Can you work these out from the model? Positions are in its coordinate system, mm. A direction names the side the tool comes from. Round coordinates to 2 decimals unless told otherwise and drop trailing zeros. Write each loop counter-clockwise with the first axis right and the second up, starting at its lowest first coordinate (ties: lowest second). Pieces come first, ordered by that corner, then holes. Notation, with made-up numbers: M 11.25,-21 L 28.25,-21 A19 cw 28.25,-16 Z; hole C 70,8.25 d11. An arc over 180 degrees is marked long. Use one line per item in the form item = value. Start each with the question number.
Autodesk Inventor part; units mm, degrees
ref_plane "YZ Plane" through (0, 0, 0) normal (1, 0, 0) x (0, 1, 0)
ref_plane "XZ Plane" through (0, 0, 0) normal (0, 1, 0) x (-1, 0, 0)
ref_plane "XY Plane" through (0, 0, 0) normal (0, 0, 1) x (1, 0, 0)
sketch "Esquisse1" plane through (0, 0, 0) normal (0, 1, 0) x (-1, 0, 0)
  line L0 (57.9966, -37.2402) -> (57.9966, 37.7598)
  circle A0 centre (52.9966, 25.0001) radius 1.75
  circle A1 centre (52.9966, 15.0001) radius 1.75
  line L1 (67, 0.0502) -> (-72, 0.0502)
  circle A2 centre (43, 25.2598) radius 1.75
  circle A3 centre (43, 15.2598) radius 1.75
  circle A4 centre (52.9966, -24.8996) radius 1.75
  circle A5 centre (52.9966, -14.8996) radius 1.75
  circle A6 centre (43, -25.1593) radius 1.75
  circle A7 centre (43, -15.1593) radius 1.75
  line L2 (0, 58.3407) -> (0, -80.6593)
  circle A8 centre (5, 31.7598) radius 2.75
  circle A9 centre (5, 22.7598) radius 1.75
  circle A10 centre (15, 32.5) radius 1.75
  circle A11 centre (15, 22.5) radius 1.75
  circle A12 centre (25, 32.5) radius 1.75
  circle A13 centre (25, 22.5) radius 1.75
  circle A14 centre (35, 22.5) radius 1.75
  circle A15 centre (5, -31.6593) radius 2.75
  circle A16 centre (5, -22.6593) radius 1.75
  circle A17 centre (15, -32.3995) radius 1.75
  circle A18 centre (15, -22.3995) radius 1.75
  circle A19 centre (25, -32.3995) radius 1.75
  circle A20 centre (25, -22.3995) radius 1.75
  circle A21 centre (35, -22.3995) radius 1.75
  line L3 (58, 10) -> (48, 10)
  line L4 (48, 10) -> (48, -10)
  line L5 (48, -10) -> (58, -10)
  line L6 (58, -10) -> (58, 10)
  line L7 (58, 10) -> (48, -10)
  line L8 (48, 10) -> (58, -10)
  line L9 (57.9966, 37.7598) -> (0, 37.7598)
  line L10 (0, -38.4609) -> (57.9966, -38.4609)
  line L11 (57.9966, -38.4609) -> (57.9966, 37.7598)
  line L12 (57.9966, 37.7598) -> (0, 37.7598)
  line L13 (0, 37.7598) -> (0, -38.4609)
  circle A22 centre (30, 0.0502) radius 11
  line L14 (42.9966, -35.3694) -> (42.9966, -32.3694)
  line L15 (42.9966, -32.3694) -> (33, -32.3694)
  line L16 (42.9966, -32.3694) -> (33, -35.5523)
  line L17 (42.9966, -35.3694) -> (33, -32.3694)
  line L18 (33, -32.3694) -> (33, -35.5523)
  line L19 (33, -35.5523) -> (42.9966, -35.3694)
  line L20 (42.9966, 31.7598) -> (42.9966, 34.7598)
  line L21 (42.9966, 34.7598) -> (32.9966, 34.7598)
  line L22 (42.9966, 34.7598) -> (32.9966, 31.7598)
  line L23 (42.9966, 31.7598) -> (32.9966, 34.7598)
  line L24 (32.9966, 34.7598) -> (32.9966, 31.7598)
  line L25 (32.9966, 31.7598) -> (42.9966, 31.7598)
  point P0 (0, 0)
  point P1 (0, 0)
  point P2 (0, 0)
  point P3 (53, 0)
  point P4 (57.9966, -10)
  point P5 (57.9966, 10)
  point P6 (38.783, -33.8694)
  point P7 (42.5405, 34.5217)
  point P8 (42.9966, -33.8694)
  point P9 (42.9966, 33.2598)
  point P10 (37.9983, -35.4609)
  dimension "d3" = 3.5
  dimension "d4" = 3.5
  dimension "d7" = 10
  dimension "d9" = 3.5
  dimension "d10" = 3.5
  dimension "d12" = 10
  dimension "d13" = 10
  dimension "d16" = 5
  dimension "d17" = 5
  dimension "d19" = 5.5
  dimension "d20" = 3.5
  dimension "d21" = 3.5
  dimension "d22" = 3.5
  dimension "d23" = 3.5
  dimension "d24" = 3.5
  dimension "d26" = 3.5
  dimension "d27" = 5
  dimension "d28" = 5
  dimension "d31" = 10
  dimension "d32" = 10
  dimension "d33" = 10
  dimension "d35" = 10
  dimension "d36" = 10
  dimension "d38" = 10
  dimension "d40" = 10
  dimension "d70" = 9
  dimension "d72" = 5
  dimension "d73" = 6
  dimension "d77" = 22
  dimension "d80" = 139
  dimension "d81" = 75
  dimension "d83" = 15
  dimension "d85" = 3
  dimension "d86" = 15
  dimension "d87" = 3
  dimension "d115" = 30
extrude "Extrusion1" add sketch "Esquisse1" along normal blind 3 contours L8 L7 L1 L0 | L5 L7 L8 | L1 L7 L0 | L4 L1 L8 L7 | L8 L1 L7 | L7 L1 L8 L3 | L4 L8 L1
sketch "Esquisse4" plane through (0, 3, 0) normal (0, 1, 0) x (1, 0, 0)
  point P0 (0, 0)
sketch "Esquisse5" plane through (0, 0, 0) normal (0, -1, 0) x (1, 0, 0)
  point P0 (0, 0)
sketch "Esquisse6" plane through (0, 0, 0) normal (0, -1, 0) x (1, 0, 0)
  point P0 (0, 0)
sketch "Esquisse7" plane through (0, 0, 0) normal (0, -1, 0) x (1, 0, 0)
  point P0 (0, 0)
sketch "Esquisse8" plane through (0, 0, 0) normal (0, -1, 0) x (1, 0, 0)
  point P0 (0, 0)
extrude "Extrusion5" cut sketch "Esquisse1" along normal blind 3 contours L8 L7 L1 L0 | L5 L7 L8 | L1 L7 L0 | L4 L1 L8 L7 | L8 L1 L7 | L7 L1 L8 L3 | L4 L8 L1 | A22 L1 | L1 A22
extrude "Extrusion7" add sketch "Esquisse1" along normal blind 3 contours L11 L10 L2 L1 A22 L4 L5 L0 | L3 L4 L1 A22 L2 L9 L0 | L17 L16 L14 | L19 L16 L17 | L16 L17 L15 | L16 L18 L17 | L23 L22 L20 | L25 L22 L23 | L22 L23 L21 | L22 L24 L23
extrude "Extrusion8" add sketch "Esquisse1" along normal blind 10 contours L23 L22 L20 | L25 L22 L23 | L22 L23 L21 | L22 L24 L23
extrude "Extrusion9" add sketch "Esquisse1" along normal blind 10 contours L17 L16 L14 | L19 L16 L17 | L16 L17 L15 | L16 L18 L17
sketch "Esquisse10" plane through (-42.9966, 3, -35.3694) normal (-0.0183, 0, -0.9998) x (-0.9998, 0, 0.0183)
  line L0 (1.2831, 0) -> (1.2831, 7)
  line L1 (1.2831, 7) -> (-10, 0)
  line L2 (-43.046, 0) -> (14.9409, 0)
  line L3 (-9.9983, 7) -> (0, 7)
  line L4 (1.2831, 0) -> (-9.9983, 7)
  circle A0 centre (-4.3576, 3.5) radius 1.75
  point P0 (-42.3423, -3)
  dimension "d108" = 3.5
sketch "Esquisse11" plane through (-42.9966, 3, 34.7598) normal (0, 0, 1) x (1, 0, 0)
  line L0 (10, 0) -> (10, 7)
  line L1 (10, 7) -> (-0.0034, 0)
  line L2 (-1.7534, 0) -> (1.7466, 0)
  line L3 (42.9966, 0) -> (-15, 0)
  line L4 (0, 0) -> (0, 7)
  line L5 (10, 0) -> (0, 7)
  circle A0 centre (4.9992, 3.5006) radius 1.75
  point P0 (42.9966, -3)
  dimension "d109" = 3.5
extrude "Extrusion10" cut sketch "Esquisse11" against normal blind 3.5 contours A0 L1 L5 | L5 L1 A0 | L1 L5 A0 | L1 A0 L5
extrude "Extrusion11" cut sketch "Esquisse10" against normal blind 3.5 contours A0 L1 L4 | L4 L1 A0 | L1 L4 A0 | A0 L4 L1
fillet "Congé10" radius 2 8 edges at (-42.9966, 10, -33.8694) (-42.9966, 3, -33.8694) (-33, 10, -33.9609) (-33, 3, -33.9609) (-32.9966, 10, 33.2598) (-32.9966, 3, 33.2598) (-42.9966, 10, 33.2598) (-42.9966, 3, 33.2598)
properties part number "toit_Impression 3D"
1. If we mould it in two halves opening along X, with no side actions, what happens to faces 1 (the face through (-29, 1, 37.76)), 2 (the face through (-16.669, 1.479, 31.974)), 3 (the face through (-32.4, 3.57, -34)), 4 (the face through (-53.9, 1.5, 23.5))? For each: pulls with the +X half, pulls with the -X half, needs draft (parallel to the pull), parting line crosses it, or undercut.
2. Will these pins go through, and if not, where does the flat tip stop? pin 1 (1.5 mm diameter, centred on x = -10.5, z = 25.5, fed in from +Y); pin 2 (1.5 mm diameter, centred on y = 6.5, z = -33, fed in from -X); pin 3 (3.5 mm diameter, centred on y = 2, z = 5.5, fed in from -X).
3. If we section it at B-B (x = -15): List the corners of the cut face in (y, z) for me, and give its area (3 significant figures).
4. Which directions (+Z, -Z, +X, -X, +Y, -Y) give clear straight access to the entire face, cutting with the end or side of a thin tool? Please do faces 5 (the face through (-32.997, 6, 33)), 6 (the face through (-53, 1, -10)), 7 (the face through (-39.746, 6.578, 33.281)).
5. If we section it at D-D (x = -5): List the corners of the cut face in (y, z) for me.
6. If we section it at C-C (z = -8): List the corners of the cut face in (x, y) for me.
7. If we section it at A-A (x = -49): List the corners of the cut face in (y, z) for me.
8. Please list where these lines run through material, in increasing order: line 1 along Z through (x, y) = (-5, 0.6); line 2 along Z through (x, y) = (-40, 9.5); line 3 along Z through (x, y) = (-25, 0.85).
Model answer:
q1.face_1 = needs draft
q1.face_2 = undercut
q1.face_3 = pulls with the +X half
q1.face_4 = undercut
q2.pin_1 = 3
q2.pin_2 = -43
q2.pin_3 = -48
q3.outline = M 0,-38.46 L 3,-38.46 L 3,-34.15 L 0,-34.15 Z; M 0,-30.65 L 3,-30.65 L 3,-24.15 L 0,-24.15 Z; M 0,-20.65 L 3,-20.65 L 3,20.75 L 0,20.75 Z; M 0,24.25 L 3,24.25 L 3,30.75 L 0,30.75 Z; M 0,34.25 L 3,34.25 L 3,37.76 L 0,37.76 Z
q3.area = 187 mm2
q4.face_5 = +Z, -Z, +X, +Y
q4.face_6 = -X, +Y, -Y
q4.face_7 = +Z
q5.outline = M 0,-38.46 L 3,-38.46 L 3,-34.41 L 0,-34.41 Z; M 0,-28.91 L 3,-28.91 L 3,-24.41 L 0,-24.41 Z; M 0,-20.91 L 3,-20.91 L 3,21.01 L 0,21.01 Z; M 0,24.51 L 3,24.51 L 3,29.01 L 0,29.01 Z; M 0,34.51 L 3,34.51 L 3,37.76 L 0,37.76 Z
q6.outline = M -48,0 L -37.5,0 L -37.5,3 L -48,3 Z; M -22.5,0 L 0,0 L 0,3 L -22.5,3 Z
q7.outline = M 0,-38.46 L 3,-38.46 L 3,-10 L 0,-10 Z; M 0,10 L 3,10 L 3,37.76 L 0,37.76 Z
q8.line_1 = -38.46 to -34.41, -28.91 to -24.41, -20.91 to 21.01, 24.51 to 29.01, 34.51 to 37.76
q8.line_2 = -35.42 to -32.37, 31.76 to 34.76
q8.line_3 = -38.46 to -34.15, -30.65 to -24.15, -20.65 to -9.75, 9.85 to 20.75, 24.25 to 30.75, 34.25 to 37.76
